Can you work these out from the model? Positions are in its coordinate system, mm. Face numbers are marked on the shaded views. A direction names the side the tool comes from. Give positions to 0.01 mm unless a question says otherwise; leave off trailing zeros. Loops run counter-clockwise (first coordinate to the right, second up) from the corner with the lowest first, then second, coordinate; pieces in that order, holes last. Notation, with made-up numbers: M -14,48.25 L -1,48.25 A35 ccw -1,81.25 Z; hole C 70,61 d9. An arc over 180 degrees is marked long. One line per item, written item: value. Start each with the question number.
from build123d import *

# Parameters (mm, degrees)
SKETCH1_R           = 13.29
BOSS_EXTRUDE1_DEPTH = 7
SKETCH2_R           = 11.54
BOSS_EXTRUDE2_DEPTH = 7.5
SKETCH3_R           = 12.16
CUT_EXTRUDE2_DEPTH  = 6
SKETCH4_R           = 10.38
CUT_EXTRUDE4_DEPTH  = 9


with BuildPart() as part:
    # Sketch1 → Boss-Extrude1 (new body)
    with BuildSketch(Plane(origin=(0, 0, 0), x_dir=(1, 0, 0), z_dir=(0, 1, 0))):
        with Locations(Location((0, 0, 0), (0, 0, 270))):
            Circle(SKETCH1_R)
    extrude(amount=BOSS_EXTRUDE1_DEPTH)

    # Sketch2 → Boss-Extrude2 (add)
    with BuildSketch(Plane(origin=(0, 7, 0), x_dir=(1, 0, 0), z_dir=(0, 1, 0))):
        with Locations(Location((0, 0, 0), (0, 0, 270))):
            Circle(SKETCH2_R)
    extrude(amount=BOSS_EXTRUDE2_DEPTH)

    # Sketch3 → Cut-Extrude2 (cut)
    with BuildSketch(Plane(origin=(0, 0, 0), x_dir=(-1, 0, 0), z_dir=(0, -1, 0))):
        with Locations(Location((0, 0, 0), (0, 0, 90))):
            Circle(SKETCH3_R)
    extrude(amount=-CUT_EXTRUDE2_DEPTH, mode=Mode.SUBTRACT)

    # Sketch4 → Cut-Extrude4 (cut)
    with BuildSketch(Plane(origin=(0, 14.5, 0), x_dir=(1, 0, 0), z_dir=(0, 1, 0))):
        with Locations(Location((0, 0, 0), (0, 0, 270))):
            Circle(SKETCH4_R)
    extrude(amount=-CUT_EXTRUDE4_DEPTH, mode=Mode.SUBTRACT)


solid = part.part
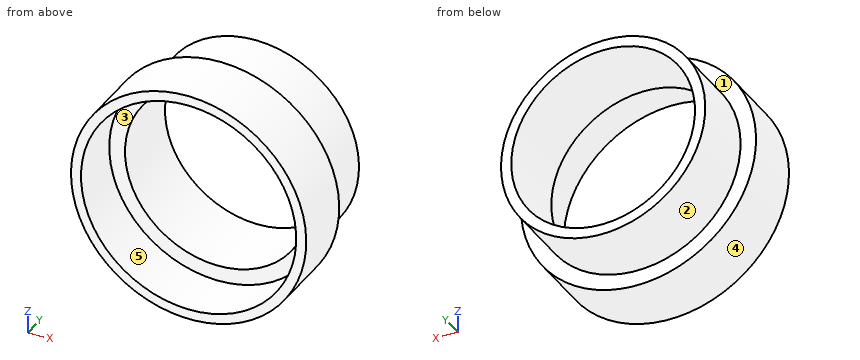
Q1. If we section it at D-D, the plane y = 3.5: Write out the boundary of the cut face in (x, z), plus the area to 3 significant figures.
Q2. Which directions (+Z, -Z, +X, -X, +Y, -Y) give clear straight access to the entire face, cutting with the end or side of a thin tool? Please do the marked faces 4 and 5.
Q3. For P1, Ø12, axis at x = 5.5, z = 1, coming from the -Y side; P2, Ø2, axis at x = -7, y = 9, coming from the +Z side; P3, Ø2, axis at y = 10.5, z = -8, coming from the +X side; P4, Ø12, axis at x = -0.5, z = -10.5, coming from the -Y side, each with a flat end and sliding along its axis, tell me the tip position at first contact or that it passes through.
Q4. If we section it at A-A, the plane z = 0: Write out the boundary of the cut face in (x, y).
Q5. If we mould it in two halves opening along Z, with no side actions, what happens to the marked faces 1, 2 and 3? For each: released by +Z, released by -Z, zero draft, split by the parting line, or undercut.
Q6. I need wall thicknesses on line 1 along X through (y, z) = (11, 0); line 2 along X through (y, z) = (3.5, 0); line 3 along Y through (x, z) = (-9.25, 7.5). Which ranges of each line are inside material? Lowest first, please.
Q7. If we section it at C-C, the plane y = 7.75: Write out the boundary of the cut face in (x, z), plus the area to 3 significant figures.
Q8. If we section it at B-B, the plane x = 0: Write out the boundary of the cut face in (y, z).
Response:
1. outline: C 0,0 d26.58; hole C 0,0 d24.32
1. area: 90.3 mm^2
2. face 4: +Y, -Y
2. face 5: -Y
3. P1: y = 6
3. P2: z = 9.86
3. P3: x = 9.17
3. P4: y = 0
4. outline: M -13.29,0 L -12.16,0 L -12.16,6 L -10.38,6 L -10.38,14.5 L -11.54,14.5 L -11.54,7 L -13.29,7 Z; M 10.38,6 L 12.16,6 L 12.16,0 L 13.29,0 L 13.29,7 L 11.54,7 L 11.54,14.5 L 10.38,14.5 Z
5. face 1: zero draft
5. face 2: split by the parting line
5. face 3: undercut
6. line 1: -11.54 to -10.38, 10.38 to 11.54
6. line 2: -13.29 to -12.16, 12.16 to 13.29
6. line 3: 6 to 7
7. outline: C 0,0 d23.08; hole C 0,0 d20.76
7. area: 79.9 mm^2
8. outline: M 0,-13.29 L 7,-13.29 L 7,-11.54 L 14.5,-11.54 L 14.5,-10.38 L 6,-10.38 L 6,-12.16 L 0,-12.16 Z; M 0,12.16 L 6,12.16 L 6,10.38 L 14.5,10.38 L 14.5,11.54 L 7,11.54 L 7,13.29 L 0,13.29 Z
